from build123d import *

# Parameters (mm, degrees)
SKETCH1_W                     = 38.1
SKETCH1_H                     = 76.2
BOSS_EXTRUDE1_DEPTH           = 2.54
M2_CLEARANCE_HOLE1_TO_DRONE_D = 2.4
M2_CLEARANCE_HOLE2_TO_PI_D    = 2.4
BOSS_EXTRUDE2_DEPTH           = 33.9852
SKETCH9_R                     = 1.50114
BOSS_EXTRUDE4_DEPTH           = 2.54
SKETCH11_W                    = 33.02
SKETCH11_H                    = 6.096
SKETCH11_R                    = 1.016
BOSS_EXTRUDE6_DEPTH           = 2.54
SKETCH12_W                    = 5.08
SKETCH12_H                    = 5.08
BOSS_EXTRUDE7_DEPTH           = 2.54
M2_CLEARANCE_HOLE1_D          = 2.4
M2_CLEARANCE_HOLE1_DEPTH      = 2.54
M2_CLEARANCE_HOLE1_TIP        = 0.721032743


with BuildPart() as part:
    # Sketch1 → Boss-Extrude1 (new body)
    with BuildSketch(Plane(origin=(0, 0, 0), x_dir=(1, 0, 0), z_dir=(0, 1, 0))):
        Rectangle(SKETCH1_W, SKETCH1_H)
    extrude(amount=BOSS_EXTRUDE1_DEPTH)

    # M2 Clearance Hole1 - to drone (through all)
    with Locations(Plane(origin=(0, 2.54, 0), x_dir=(1, 0, 0), z_dir=(0, 1, 0))):
        with Locations((-13.97, 0), (13.97, 0)):
            Hole(M2_CLEARANCE_HOLE1_TO_DRONE_D / 2)

    # M2 Clearance Hole2 - to Pi (through all)
    with Locations(Plane(origin=(0, 2.54, 0), x_dir=(1, 0, 0), z_dir=(0, 1, 0))):
        with Locations((-5.69976, 23.50008), (5.69976, 23.50008), (5.69976, -23.50008), (-5.69976, -23.50008)):
            Hole(M2_CLEARANCE_HOLE2_TO_PI_D / 2)

    # Sketch7 → Boss-Extrude2 (add)
    with BuildSketch(Plane(origin=(0, 2.54, 0), x_dir=(1, 0, 0), z_dir=(0, 1, 0))):
        Polygon((-19.05, -38.1), (-19.05, -35.56), (-19.05, 38.1), (-16.51, 38.1), (-16.51, -35.56), (16.51, -35.56), (16.51, 38.1), (19.05, 38.1), (19.05, -38.1), align=None)
    extrude(amount=BOSS_EXTRUDE2_DEPTH)

    # Sketch11 → Boss-Extrude6 (add)
    with BuildSketch(Plane(origin=(0, 19.5326, 0), x_dir=(1, 0, 0), z_dir=(0, 1, 0))):
        with Locations((0, -32.512)):
            Rectangle(SKETCH11_W, SKETCH11_H)
        with Locations((-6.985, -31.75)):
            Circle(SKETCH11_R, mode=Mode.SUBTRACT)
        with Locations((6.985, -31.75)):
            Circle(SKETCH11_R, mode=Mode.SUBTRACT)
    extrude(amount=-BOSS_EXTRUDE6_DEPTH)



with BuildPart() as body_2:
    # Sketch9 → Boss-Extrude4 (new body)
    with BuildSketch(Plane(origin=(0, 0, -38.1), x_dir=(-1, 0, 0), z_dir=(0, 0, -1))):
        Polygon((-11.43, 8.89), (11.43, 8.89), (11.43, 36.5252), (16.51, 36.5252), (16.51, 2.54), (-16.51, 2.54), (-16.51, 36.5252), (-11.43, 36.5252), align=None)
        with Locations((-10.31494, 5.715)):
            Circle(SKETCH9_R, mode=Mode.SUBTRACT)
        with Locations((10.31494, 5.715)):
            Circle(SKETCH9_R, mode=Mode.SUBTRACT)
    extrude(amount=-BOSS_EXTRUDE4_DEPTH)


with BuildPart() as part_1:
    add(part.part)

    add(body_2.part)  # Boss-Extrude7 merges body 2
    # Sketch12 → Boss-Extrude7 (add)
    with BuildSketch(Plane(origin=(0, 36.5252, 0), x_dir=(1, 0, 0), z_dir=(0, 1, 0))):
        with Locations((-13.97, -33.02)):
            Rectangle(SKETCH12_W, SKETCH12_H)
        with Locations((13.97, -33.02)):
            Rectangle(SKETCH12_W, SKETCH12_H)
        with Locations((13.97, 33.02)):
            Rectangle(SKETCH12_W, SKETCH12_H)
        with Locations((-13.97, 33.02)):
            Rectangle(SKETCH12_W, SKETCH12_H)
    extrude(amount=-BOSS_EXTRUDE7_DEPTH)

    # M2 Clearance Hole1
    with Locations(Plane(origin=(0, 36.5252, 0), x_dir=(1, 0, 0), z_dir=(0, 1, 0))):
        with Locations((-13.97, 33.02), (13.97, 33.02), (13.97, -33.02), (-13.97, -33.02)):
            Hole(M2_CLEARANCE_HOLE1_D / 2, depth=M2_CLEARANCE_HOLE1_DEPTH)
            with Locations((0, 0, -(M2_CLEARANCE_HOLE1_DEPTH + M2_CLEARANCE_HOLE1_TIP / 2))):  # 118° drill point
                Cone(0, M2_CLEARANCE_HOLE1_D / 2, M2_CLEARANCE_HOLE1_TIP, mode=Mode.SUBTRACT)


solid = part_1.part
The listing builds one solid part. Answer for the finished solid, in the listing's coordinates (mm). A direction names the side the tool comes from. Round coordinates to 2 decimals unless told otherwise and drop trailing zeros. Write each loop counter-clockwise with the first axis right and the second up, starting at its lowest first coordinate (ties: lowest second). Pieces come first, ordered by that corner, then holes. Notation, with made-up numbers: (-40, 30) - (-8, 30) arc R27 cw to (-8, 61) - close; hole circle Ø7 at (70, 74.25). An arc over 180 degrees is marked (long way). Use a Markdown table: item, result. Add a question column.
1. Consider line 1 (X direction, y = 35, z = -33); line 2 (X direction, y = 13, z = -23); line 3 (Z direction, x = -12.5, y = 11.5). Determine where each line is inside the solid, lowest interval first.
2. The part is cut by section A-A (x = 13.97). Write down the section's boundary in (y, z).
3. Flat-ended cylindrical pins translate along their axes: P1, Ø5, axis at x = 6.5, z = 31.5, coming from the +Y side; P2, Ø6, axis at x = 1, z = 9.5, coming from the +Y side; P3, Ø7, axis at x = 5.5, y = 13, coming from the -Z side. Find the tip coordinate at first contact, or state that the pin passes through.
4. For a pull along X with two mould halves and no side action, classify faces 4 (the face through (19.05, 18, -1)), 5 (the face through (-17, 36.525, 5)), 6 (the face through (-12.77, 1.25, -0.05)) as +X half, -X half, draft (parallel to the pull), parting line (faces both ways), or undercut.
5. A tool of negligible diameter and unlimited length cuts with its end or side. For faces 1 (the face through (-15, 33.985, -32)), 2 (the face through (14, 35, 30.48)), 3 (the face through (5.146, 1.252, -22.435)), from which of +Z, -Z, +X, -X, +Y, -Y can it reach the whole face along a straight path? Write none if from no direction.
6. The part is cut by section C-C (y = 30). Write down the section's boundary in (x, z), and give its area (3 significant figures).
7. The part is cut by section B-B (z = -33.02). Write down the section's boundary in (x, y).
8. The part is cut by section D-D (z = -21). Write down the section's boundary in (x, y), and give its area (3 significant figures).
Reported:
| question | item | result |
|---|---|---|
| 1 | line 1 | -19.05 to -15.17, -12.77 to -11.43, 11.43 to 12.77, 15.17 to 19.05 |
| 1 | line 2 | -19.05 to -16.51, 16.51 to 19.05 |
| 1 | line 3 | -38.1 to -35.56, 35.56 to 38.1 |
| 2 | outline | (0, -38.1) - (36.53, -38.1) - (36.53, -34.22) - (33.99, -34.22) - (33.99, -35.56) - (2.54, -35.56) - (2.54, -1.2) - (0, -1.2) - close; (0, 1.2) - (2.54, 1.2) - (2.54, 35.56) - (16.99, 35.56) - (16.99, 29.46) - (19.53, 29.46) - (19.53, 35.56) - (33.99, 35.56) - (33.99, 34.22) - (36.53, 34.22) - (36.53, 38.1) - (0, 38.1) - close; (33.99, -31.82) - (36.53, -31.82) - (36.53, -30.48) - (33.99, -30.48) - close; (33.99, 30.48) - (36.53, 30.48) - (36.53, 31.82) - (33.99, 31.82) - close |
| 3 | P1 | y = 19.53 |
| 3 | P2 | y = 2.54 |
| 3 | P3 | z = 35.56 |
| 4 | face 4 | +X half |
| 4 | face 5 | draft |
| 4 | face 6 | undercut |
| 5 | face 1 | none |
| 5 | face 2 | +Y |
| 5 | face 3 | +Y, -Y |
| 6 | outline | (-19.05, -38.1) - (-11.43, -38.1) - (-11.43, -35.56) - (-16.51, -35.56) - (-16.51, 35.56) - (16.51, 35.56) - (16.51, -35.56) - (11.43, -35.56) - (11.43, -38.1) - (19.05, -38.1) - (19.05, 38.1) - (-19.05, 38.1) - close |
| 6 | area | 497 mm^2 |
| 7 | outline | (-19.05, 0) - (19.05, 0) - (19.05, 36.53) - (15.17, 36.53) - (15.17, 33.99) - (16.51, 33.99) - (16.51, 2.54) - (-16.51, 2.54) - (-16.51, 33.99) - (-15.17, 33.99) - (-15.17, 36.53) - (-19.05, 36.53) - close; (-12.77, 33.99) - (-11.43, 33.99) - (-11.43, 36.53) - (-12.77, 36.53) - close; (11.43, 33.99) - (12.77, 33.99) - (12.77, 36.53) - (11.43, 36.53) - close |
| 8 | outline | (-19.05, 0) - (19.05, 0) - (19.05, 36.53) - (16.51, 36.53) - (16.51, 2.54) - (-16.51, 2.54) - (-16.51, 36.53) - (-19.05, 36.53) - close |
| 8 | area | 269 mm^2 |
